Could you check a few things on this drawing? It's one solid part, dimensions in mm from its lowest x, y, z. A direction names the side the tool comes from. Coordinates: 2 decimals unless noted, no trailing zeros. Order: outer loops, then holes, each group sorted by start corner. A loop starts at its lowest first (then second) coordinate and runs counter-clockwise, first axis right, second up. Notation, with made-up numbers: (-24, 38.5) - (24, 38.5) arc R11 ccw to (24, 50.5) - close; hole circle Ø5 at (-31.5, -6.75). An arc over 180 degrees is marked (long way). Return JSON: item names as keys, results as strings. Group by question number.
1) Imagine slicing it at D-D (y = 143). Write out the boundary of the cut face in (x, z), and give its area (3 significant figures).
2) If we mould it in two halves opening along Y, with no side actions, what happens to the marked faces 1, 2 and 3? For each: pulls with the +Y half, pulls with the -Y half, needs draft (parallel to the pull), parting line crosses it, or undercut.
3) Imagine slicing it at C-C (x = 4). Write out the boundary of the cut face in (y, z).
4) Imagine slicing it at B-B (x = 19.05). Write out the boundary of the cut face in (y, z).
5) Imagine slicing it at A-A (z = 9.5). Write out the boundary of the cut face in (x, y).
6) Which directions (+Z, -Z, +X, -X, +Y, -Y) give clear straight access to the entire face, cutting with the end or side of a thin tool? Please do the marked faces 4 and 5.
7) If I drill on line 1 along Y through (x, z) = (19.05, 1.55); line 2 along Y through (x, z) = (29, 14.5); line 3 along Y through (x, z) = (10.5, 0.75) (1 decimal), over which ranges is the centre line in solid material (lowest first)?
8) For pin 1 Ø16.5 at (x, y) = (19.05, 107.696) entering from -Z; pin 2 Ø6 at (y, z) = (95.5, 6) entering from +X (1 decimal); pin 3 Ø1 at (x, y) = (22.5, 129.5) entering from +Z; pin 4 Ø5 at (y, z) = (121, 1.5) entering from +X, each with a flat end and sliding along its axis, tell me the tip position at first contact or that it passes through.
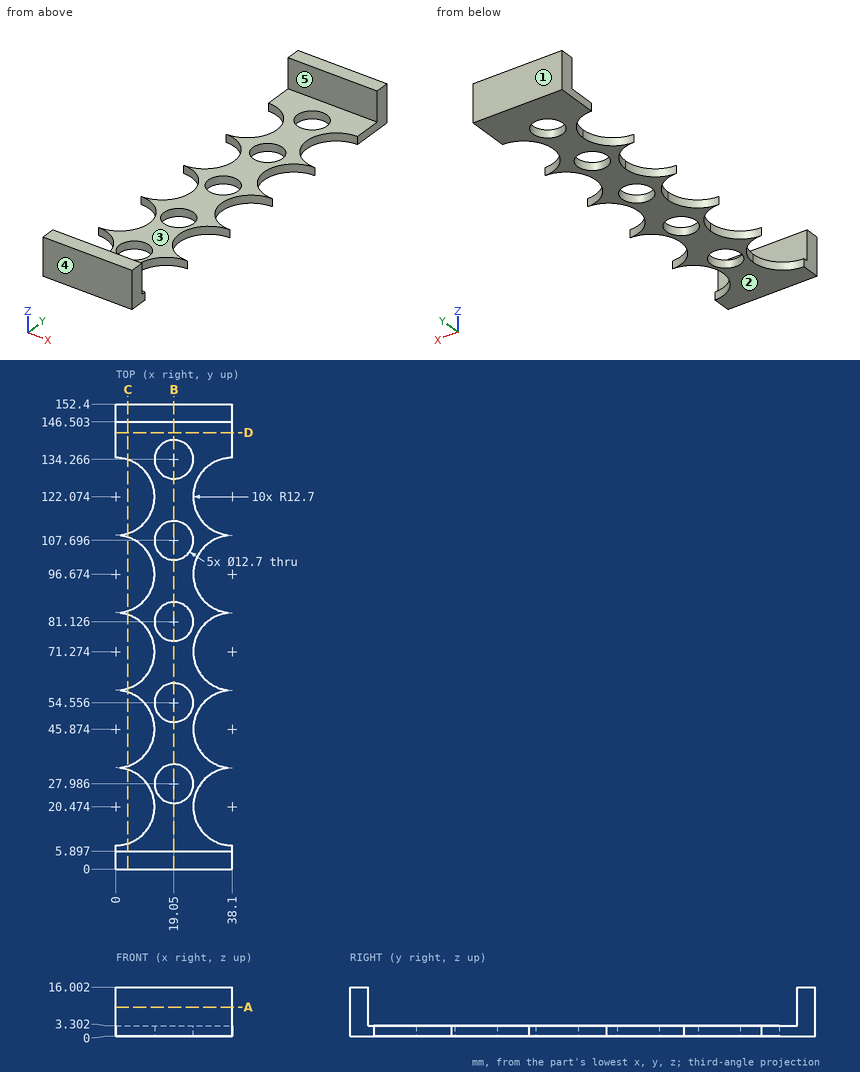
Calculated:
{
 "1": {"outline": "(0, 0) - (38.1, 0) - (38.1, 3.3) - (0, 3.3) - close", "area": "126 mm2"},
 "2": {"face 1": "pulls with the +Y half", "face 2": "needs draft", "face 3": "undercut"},
 "3": {"outline": "(0, 0) - (8.42, 0) - (8.42, 3.3) - (5.9, 3.3) - (5.9, 16) - (0, 16) - close; (32.53, 0) - (33.82, 0) - (33.82, 3.3) - (32.53, 3.3) - close; (57.93, 0) - (59.22, 0) - (59.22, 3.3) - (57.93, 3.3) - close; (83.33, 0) - (84.62, 0) - (84.62, 3.3) - (83.33, 3.3) - close; (108.73, 0) - (110.02, 0) - (110.02, 3.3) - (108.73, 3.3) - close; (134.13, 0) - (152.4, 0) - (152.4, 16) - (146.5, 16) - (146.5, 3.3) - (134.13, 3.3) - close"},
 "4": {"outline": "(0, 0) - (21.64, 0) - (21.64, 3.3) - (5.9, 3.3) - (5.9, 16) - (0, 16) - close; (34.34, 0) - (48.21, 0) - (48.21, 3.3) - (34.34, 3.3) - close; (60.91, 0) - (74.78, 0) - (74.78, 3.3) - (60.91, 3.3) - close; (87.48, 0) - (101.35, 0) - (101.35, 3.3) - (87.48, 3.3) - close; (114.05, 0) - (127.92, 0) - (127.92, 3.3) - (114.05, 3.3) - close; (140.62, 0) - (152.4, 0) - (152.4, 16) - (146.5, 16) - (146.5, 3.3) - (140.62, 3.3) - close"},
 "5": {"outline": "(0, 0) - (38.1, 0) - (38.1, 5.9) - (0, 5.9) - close; (0, 146.5) - (38.1, 146.5) - (38.1, 152.4) - (0, 152.4) - close"},
 "6": {"face 4": "+Z, -Z, +X, -X, -Y", "face 5": "+Z, +X, -X"},
 "7": {"line 1": "0 to 21.64, 34.34 to 48.21, 60.91 to 74.78, 87.48 to 101.35, 114.05 to 127.92, 140.62 to 152.4", "line 2": "0 to 5.9, 146.5 to 152.4", "line 3": "0 to 13.3, 27.6 to 38.7, 53 to 64.1, 78.4 to 89.5, 103.8 to 114.9, 129.2 to 152.4"},
 "8": {"pin 1": "z = 0", "pin 2": "x = 25.6", "pin 3": "z = 3.3", "pin 4": "x = 25.91"}
}
